Geometry check sheet. Reference: the model listing, model coordinates, mm. Face numbers are marked on the shaded views. A direction names the side the tool comes from. Coordinates: 2 decimals unless noted, no trailing zeros. Write each loop counter-clockwise with the first axis right and the second up, starting at its lowest first coordinate (ties: lowest second). Pieces come first, ordered by that corner, then holes. Notation, with made-up numbers: M 74.5,-24 L 131.5,-24 A21 ccw 131.5,7 Z; hole C 11.5,65.25 d2. An arc over 180 degrees is marked long. Write each question's results on one line, items separated by ' | '.
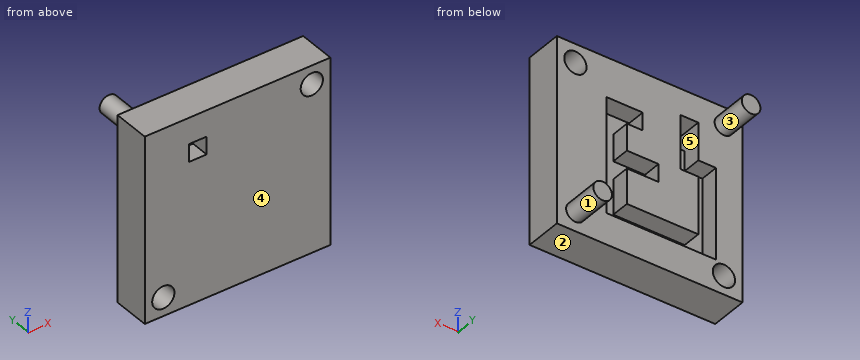
```python
from build123d import *

# Parameters (mm, degrees)
F0_R          = 3
F0_R_2        = 2.5
F1_DEPTH      = 5
F0_W          = 4.7752
F0_H          = 4.7752
F2_DEPTH      = 5
F3_DEPTH      = 15
F3_DEPTH_BACK = 5


with BuildPart() as f1:
    # F0 (on Front) → F1 (new body, symmetric)
    with BuildSketch(Plane.XZ):
        Polygon((-25, -25), (25, -25), (25, 25), (-13.09502, 25), (-25, 25), align=None)
        with Locations((-20, -20)):
            Circle(F0_R, mode=Mode.SUBTRACT)
        with Locations((20, -20)):
            Circle(F0_R_2, mode=Mode.SUBTRACT)
        Polygon((-13.09502, 13.21694), (-13.09502, 17.97944), (-8.33252, 17.97944), (-8.33252, 13.21694), (-8.33252, 3.5414441053), (-13.09502, 3.5414441053), (-13.09502, -11.8404025305), (-4.4399380628, -11.8404025305), (6.1322724736, -11.8404025305), (6.1322724736, -2.3876), (2.3876, -2.3876), (-2.3876, -2.3876), (-2.3876, 2.3876), (2.3876, 2.3876), (6.1322724736, 2.3876), (6.1322724736, 9.5728570595), (1.8619408365, 9.5728570595), (1.8619408365, 14.3480570595), (8.9338924736, 14.3480570595), (11.5732288948, 14.3480570595), (11.5732288948, 13.8279201027), (11.5732288948, 9.2561525788), (11.5732288948, 2.3876), (11.5732288948, -2.3876), (11.5732288948, -16.6029025305), (-17.85752, -16.6029025305), (-17.85752, 3.5414441053), (-17.85752, 7.8989091825), (-13.09502, 7.8989091825), align=None, mode=Mode.SUBTRACT)
        with Locations((-20, 20)):
            Circle(F0_R_2, mode=Mode.SUBTRACT)
        with Locations((20, 20)):
            Circle(F0_R, mode=Mode.SUBTRACT)
    extrude(amount=F1_DEPTH, both=True)

    # F0 (on Front) → F2 (join)
    with BuildSketch(Plane.XZ):
        Polygon((-8.33252, 13.21694), (-13.09502, 13.21694), (-13.09502, 7.8989091825), (-17.85752, 7.8989091825), (-17.85752, 3.5414441053), (-17.85752, -16.6029025305), (11.5732288948, -16.6029025305), (11.5732288948, -2.3876), (11.5732288948, 2.3876), (11.5732288948, 9.2561525788), (11.5732288948, 13.8279201027), (11.5732288948, 14.3480570595), (8.9338924736, 14.3480570595), (1.8619408365, 14.3480570595), (1.8619408365, 9.5728570595), (6.1322724736, 9.5728570595), (6.1322724736, 2.3876), (2.3876, 2.3876), (2.3876, -2.3876), (6.1322724736, -2.3876), (6.1322724736, -11.8404025305), (-4.4399380628, -11.8404025305), (-13.09502, -11.8404025305), (-13.09502, 3.5414441053), (-8.33252, 3.5414441053), align=None)
        Rectangle(F0_W, F0_H)
    extrude(amount=F2_DEPTH)

    # F0 (on Front) → F3 (join, two sides)
    with BuildSketch(Plane.XZ) as f3_sk:
        with Locations((-20, 20)):
            Circle(F0_R_2)
        with Locations((20, -20)):
            Circle(F0_R_2)
    extrude(amount=-F3_DEPTH)
    extrude(f3_sk.sketch, amount=F3_DEPTH_BACK)


solid = f1.part
```
Q1. Access from +Z, -Z, +X, -X, +Y, -Y to the whole of each face (thin tool, end or side, straight path). Record for the marked faces 1 and 2.
Geometry check:
face 1: +Y | face 2: -Z, +X, -X, +Y, -Y
Q2. Sectioned sample at B-B on x = -20. Record the cut outline in (y, z), and give its area (3 significant figures).
Geometry check:
outline: M -5,-25 L 5,-25 L 5,-23 L -5,-23 Z; M -5,-17 L 5,-17 L 5,17.5 L 15,17.5 L 15,22.5 L 5,22.5 L 5,25 L -5,25 Z | area: 490 mm2
Q3. Sectioned sample at A-A on z = -20. Record the cut outline in (x, y), and give its area (3 significant figures).
Geometry check:
outline: M -25,-5 L -23,-5 L -23,5 L -25,5 Z; M -17,-5 L 25,-5 L 25,5 L 22.5,5 L 22.5,15 L 17.5,15 L 17.5,5 L -17,5 Z | area: 490 mm2
Q4. Mould release check, pull along Z, two halves, no side actions. Record for the marked faces 3, 4 and 5: pulls with the +Z half, pulls with the -Z half, needs draft (parallel to the pull), parting line crosses it, or undercut.
Geometry check:
face 3: parting line crosses it | face 4: needs draft | face 5: undercut
Q5. Sectioned sample at D-D on z = 12. Record the cut outline in (x, y).
Geometry check:
outline: M -25,-5 L 25,-5 L 25,5 L 11.57,5 L 11.57,0 L 1.86,0 L 1.86,5 L -8.33,5 L -8.33,0 L -13.1,0 L -13.1,5 L -25,5 Z
Q6. Scan lines: probe 1 along Z at (x, y) = (0.5, 4); probe 2 along X at (y, z) = (2, 2.5); probe 3 along Z at (x, y) = (-20, 0.75). Record each from-to range of solid material in increasing order.
Geometry check:
probe 1: z = -25 to -16.6, -11.84 to -2.39, 2.39 to 25 | probe 2: x = -25 to -17.86, -13.1 to 6.13, 11.57 to 25 | probe 3: z = -25 to -23, -17 to 25
Q7. Sectioned sample at C-C on y = 1. Record the cut outline in (x, z), and give its area (3 significant figures).
Geometry check:
outline: M -25,-25 L 25,-25 L 25,25 L -25,25 Z; hole C -20,-20 d6; hole M -17.86,-16.6 L 11.57,-16.6 L 11.57,14.35 L 1.86,14.35 L 1.86,9.57 L 6.13,9.57 L 6.13,2.39 L -2.39,2.39 L -2.39,-2.39 L 6.13,-2.39 L 6.13,-11.84 L -13.1,-11.84 L -13.1,3.54 L -8.33,3.54 L -8.33,17.98 L -13.1,17.98 L -13.1,7.9 L -17.86,7.9 Z; hole C 20,20 d6 | area: 1,940 mm2
